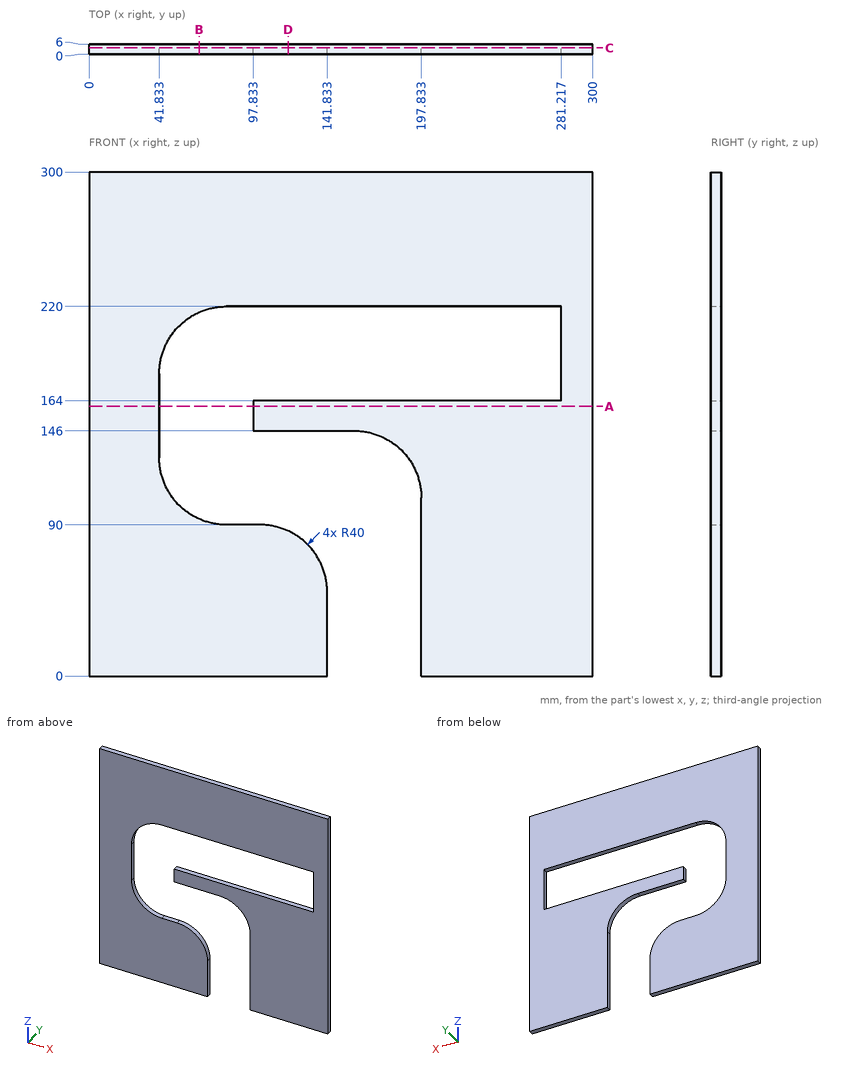
Verification items for this drawing (mm, ordinates from the low corner). Coordinates: 2 decimals unless noted, no trailing zeros. Order: outer loops, then holes, each group sorted by start corner. A loop starts at its lowest first (then second) coordinate and runs counter-clockwise, first axis right, second up. Notation, with made-up numbers: (65, -36.75) - (119, -36.75) arc R26 cw to (119, -14.75) - close; hole circle Ø4 at (86.25, 15). An arc over 180 degrees is marked (long way). Use one line per item in the form item = value.
1. Section check B-B (x = 65.5). Record the boundary of the cut face in (y, z).
Here are the results:
outline = (0, 0) - (6, 0) - (6, 93.49) - (0, 93.49) - close; (0, 216.51) - (6, 216.51) - (6, 300) - (0, 300) - close
2. Scan lines: line 1 (X direction, y = 1.05, z = 178); line 2 (Z direction, x = 268, y = 4.5); line 3 (Z direction, x = 117.5, y = 4.15) (1 decimal). Record each from-to range of solid material in increasing order.
Here are the results:
line_1 = 0 to 41.83, 281.22 to 300
line_2 = 0 to 164, 220 to 300
line_3 = 0 to 86.8, 146 to 164, 220 to 300
3. Section check D-D (x = 118.5). Record the boundary of the cut face in (y, z), then the cut area to 3 significant figures.
Here are the results:
outline = (0, 0) - (6, 0) - (6, 86.36) - (0, 86.36) - close; (0, 146) - (6, 146) - (6, 164) - (0, 164) - close; (0, 220) - (6, 220) - (6, 300) - (0, 300) - close
area = 1,110 mm²
4. Gauge pin test, flat end, axial feed: pin 1 (3 mm diameter, centred on x = 147.5, y = 4, fed in from -Z). Record the tip position at first contact, or that the pin passes through.
Here are the results:
pin_1 = 146
5. Section check C-C (y = 3.75). Record the boundary of the cut face in (x, z).
Here are the results:
outline = (0, 0) - (141.83, 0) - (141.83, 50) arc R40 ccw to (101.83, 90) - (81.83, 90) arc R40 cw to (41.83, 130) - (41.83, 180) arc R40 cw to (81.83, 220) - (281.22, 220) - (281.22, 164) - (97.83, 164) - (97.83, 146) - (157.83, 146) arc R40 cw to (197.83, 106) - (197.83, 0) - (300, 0) - (300, 300) - (0, 300) - close
6. Section check A-A (z = 160.5). Record the boundary of the cut face in (x, y).
Here are the results:
outline = (0, 0) - (41.83, 0) - (41.83, 6) - (0, 6) - close; (97.83, 0) - (300, 0) - (300, 6) - (97.83, 6) - close
